Geometry check sheet. Reference: the model listing, model coordinates, mm. A direction names the side the tool comes from. Round coordinates to 2 decimals unless told otherwise and drop trailing zeros. Order: outer loops, then holes, each group sorted by start corner. A loop starts at its lowest first (then second) coordinate and runs counter-clockwise, first axis right, second up. Notation, with made-up numbers: (47.25, 89.25) - (77.25, 89.25) arc R20 cw to (77.25, 124.25) - close; hole circle Ø5 at (5, -15.75). An arc over 180 degrees is marked (long way). Use a Markdown table: item, result. Add a question column.
(1) Gauge pin test, flat ends, axial feed: P1, Ø5, axis at x = 9, y = -5, coming from the -Z side; P2, Ø12, axis at x = 3.5, z = 113.5, coming from the +Y side; P3, Ø3, axis at x = 11, z = 89.5, coming from the -Y side; P4, Ø10, axis at x = 11.5, z = 24.5, coming from the +Y side. Record the tip position at first contact, or that the pin passes through.
(2) Thickness scan on line 1 along X through (y, z) = (6, 1.8); line 2 along Y through (x, z) = (21, 1.55); line 3 along X through (y, z) = (-6, 4). Record the ranges inside material, lowest first. Write a range as [from, to].
(3) Section check A-A on x = 9. Record the boundary of the cut face in (y, z), then the cut area to 3 significant figures.
(4) Access from +Z, -Z, +X, -X, +Y, -Y to the whole of each face (thin tool, end or side, straight path). Record for faces 1 (the face through (21, 6, 5.5)), 2 (the face through (9, 6, -5)), 3 (the face through (20.957, 13.628, 116.576)).
(5) Section check B-B on y = -6. Record the boundary of the cut face in (x, z).
(6) Section check D-D on y = 1. Record the boundary of the cut face in (x, z).
(7) Section check C-C on z = 44. Record the boundary of the cut face in (x, y).
(8) Mould release check, pull along X, two halves, no side actions. Record for faces 4 (the face through (9, -6, 5.5)), 5 (the face through (11.77, 15.06, 124.01)), 6 (the face through (20.972, 28.482, 122.344)): released by +X, released by -X, zero draft, split by the parting line, or undercut.
```python
from build123d import *

# Parameters (mm, degrees)
F1_DEPTH  = 30
F2_R      = 3
F3_DEPTH  = 5
F4_SIZE   = 1
F5_R      = 3
F6_DEPTH  = 5
F7_SIZE   = 1
F8_R      = 3.05
F9_DEPTH  = 5.5
F10_R     = 3.05
F11_DEPTH = 5.5


with BuildPart() as f1:
    # F0 (on Right) → F1 (new body)
    with BuildSketch(Plane.YZ):
        with BuildLine():
            ThreePointArc((7.0121934131, 124.8373523139), (-9.4548298495, 63.3815848484), (-15, 0))
            Line((-15, 0), (15, 0))
            ThreePointArc((15, 0), (20.0894027409, 58.1721395184), (35.2029720367, 114.5767480141))
            Line((35.2029720367, 114.5767480141), (7.0121934131, 124.8373523139))
        make_face()
    extrude(amount=F1_DEPTH)

    # F2 (on face) → F3 (join)
    with BuildSketch(Plane(origin=(0, 40.9422224542, 112.4878316951), x_dir=(1, 0, 0), z_dir=(0, 0.3420201433, 0.9396926208))):
        with Locations((9, -27.1075827249)):
            Circle(F2_R)
        with Locations((21, -15.1075827249)):
            Circle(F2_R)
    extrude(amount=F3_DEPTH)

    # F4
    f4_edges = [f1.edges().sort_by_distance(p)[0] for p in [
        (6, 17.179528, 126.457634),
        (18, 28.455839, 122.353392),
    ]]
    chamfer(f4_edges, length=F4_SIZE)

    # F5 (on face) → F6 (join)
    with BuildSketch(Plane(origin=(0, 0, 0), x_dir=(1, 0, 0), z_dir=(0, 0, -1))):
        with Locations((9, -6)):
            Circle(F5_R)
        with Locations((21, 6)):
            Circle(F5_R)
    extrude(amount=F6_DEPTH)

    # F7
    f7_edges = [f1.edges().sort_by_distance(p)[0] for p in [
        (6, 6, -5),
        (18, -6, -5),
    ]]
    chamfer(f7_edges, length=F7_SIZE)

    # F8 (on face) → F9 (cut)
    with BuildSketch(Plane(origin=(0, 40.9422224542, 112.4878316951), x_dir=(1, 0, 0), z_dir=(0, 0.3420201433, 0.9396926208))):
        with Locations((9, -15.1075827249)):
            Circle(F8_R)
        with Locations((21, -27.1075827249)):
            Circle(F8_R)
    extrude(amount=-F9_DEPTH, mode=Mode.SUBTRACT)

    # F10 (on face) → F11 (cut)
    with BuildSketch(Plane(origin=(0, 0, 0), x_dir=(1, 0, 0), z_dir=(0, 0, -1))):
        with Locations((9, 6)):
            Circle(F10_R)
        with Locations((21, -6)):
            Circle(F10_R)
    extrude(amount=-F11_DEPTH, mode=Mode.SUBTRACT)


solid = f1.part
```
Check sheet entries:
| question | item | result |
|---|---|---|
| 1 | P1 | stops at z = 0 |
| 1 | P2 | stops at y = 35.2 |
| 1 | P3 | stops at y = -4.23 |
| 1 | P4 | stops at y = 16.3 |
| 2 | line 1 | x = [0, 17.95], [24.05, 30] |
| 2 | line 2 | y = [-15, 2.95], [9.05, 15] |
| 2 | line 3 | x = [0, 5.95], [12.05, 30] |
| 3 | outline | (-15, 0) - (-9.05, 0) - (-9.05, 5.5) - (-2.95, 5.5) - (-2.95, 0) - (3, 0) - (3, -4) - (4, -5) - (8, -5) - (9, -4) - (9, 0) - (15, 0) arc R335 cw to (35.2, 114.58) - (29.61, 116.61) - (27.73, 111.44) - (22, 113.53) - (23.88, 118.7) - (18.29, 120.73) - (19.66, 124.49) - (19.06, 125.77) - (15.3, 127.14) - (14.02, 126.54) - (12.65, 122.79) - (7.01, 124.84) arc R365 ccw to start |
| 3 | area | 3,660 mm2 |
| 4 | face 1 | -Z |
| 4 | face 2 | -Z, +X, -X, +Y, -Y |
| 4 | face 3 | none |
| 5 | outline | (0, 0) - (5.95, 0) - (5.95, 5.5) - (12.05, 5.5) - (12.05, 0) - (18, 0) - (18, -4) - (19, -5) - (23, -5) - (24, -4) - (24, 0) - (30, 0) - (30, 80.55) - (0, 80.55) - close |
| 6 | outline | (0, 0) - (30, 0) - (30, 106.88) - (0, 106.88) - close |
| 7 | outline | (0, -12.34) - (30, -12.34) - (30, 17.9) - (0, 17.9) - close |
| 8 | face 4 | undercut |
| 8 | face 5 | split by the parting line |
| 8 | face 6 | zero draft |
